```python
from build123d import *

# Parameters (mm, degrees)
F0_W     = 116.948664
F0_H     = 61.326738
F0_W_2   = 104.968556
F0_H_2   = 48.77615
F1_DEPTH = 50.8
F2_W     = 55.336682
F2_H     = 18.995669
F3_DEPTH = 76.2
F4_R     = 6.426074
F5_DEPTH = 177.8


with BuildPart() as f1:
    # F0 (on Top) → F1 (new body)
    with BuildSketch(Plane.XY):
        with Locations((3.137648, -3.137646)):
            Rectangle(F0_W, F0_H)
        with Locations((3.708128, -3.137648)):
            Rectangle(F0_W_2, F0_H_2, mode=Mode.SUBTRACT)
    extrude(amount=F1_DEPTH)

    # F2 (on face) → F3 (cut)
    with BuildSketch(Plane.XZ.offset(33.801015)):
        with Locations((2.281924, 41.302166)):
            Rectangle(F2_W, F2_H)
    extrude(amount=-F3_DEPTH, mode=Mode.SUBTRACT)

    # F4 (on face) → F5 (cut)
    with BuildSketch(Plane.YZ.offset(61.61198)):
        with Locations((-3.137646, 25.4)):
            Circle(F4_R)
    extrude(amount=-F5_DEPTH, mode=Mode.SUBTRACT)


solid = f1.part
```
For this review, take the finished solid that the model builds, in its own axes (mm). A direction names the side the tool comes from. Round coordinates to 2 decimals unless told otherwise and drop trailing zeros. Order: outer loops, then holes, each group sorted by start corner. A loop starts at its lowest first (then second) coordinate and runs counter-clockwise, first axis right, second up.
Q1. Mouldability with a two-part tool opening along Y and no side actions: class faces 4 (the cylindrical face through (58.94, -3.97, 31.77)), 5 (the flat face through (2, -31, 31.804)), 6 (the flat face through (3, -27.526, 19)), 7 (the flat face through (2, -33.801, 19)) as pulls with the +Y half, pulls with the -Y half, needs draft (parallel to the pull), parting line crosses it, or undercut.
Findings below:
face 4: undercut
face 5: needs draft
face 6: undercut
face 7: pulls with the -Y half
Q2. We need section A-A, the plane x = -8. Give the boundary of the cut face in (y, z).
Findings below:
outline: (-33.8, 0) - (-27.53, 0) - (-27.53, 31.8) - (-33.8, 31.8) - close; (21.25, 0) - (27.53, 0) - (27.53, 31.8) - (21.25, 31.8) - close
Q3. Insertion check: P1, Ø7, axis at x = 3.5, y = -31, coming from the +Z side. The pin has a flat end and moves straight along its axis. Give the tip position at first contact, or say it passes through.
Findings below:
P1: stops at z = 31.8
Q4. We need section C-C, the plane y = -2. Give the boundary of the cut face in (x, z), plus the area to 3 significant figures.
Findings below:
outline: (-55.34, 0) - (-48.78, 0) - (-48.78, 19.08) - (-55.34, 19.08) - close; (-55.34, 31.72) - (-48.78, 31.72) - (-48.78, 50.8) - (-55.34, 50.8) - close; (56.19, 0) - (61.61, 0) - (61.61, 19.08) - (56.19, 19.08) - close; (56.19, 31.72) - (61.61, 31.72) - (61.61, 50.8) - (56.19, 50.8) - close
area: 457 mm2
Q5. We need section B-B, the plane z = 35. Give the boundary of the cut face in (x, y), plus the area to 3 significant figures.
Findings below:
outline: (-55.34, -33.8) - (-25.39, -33.8) - (-25.39, -27.53) - (-48.78, -27.53) - (-48.78, 21.25) - (-25.39, 21.25) - (-25.39, 27.53) - (-55.34, 27.53) - close; (29.95, -33.8) - (61.61, -33.8) - (61.61, 27.53) - (29.95, 27.53) - (29.95, 21.25) - (56.19, 21.25) - (56.19, -27.53) - (29.95, -27.53) - close
area: 1,360 mm2
Q6. Wall thickness on line 1 (X direction, y = 24.5, z = 49); line 2 (Y direction, x = -26, z = 38); line 3 (X direction, y = 10, z = 8): over which ranges is each line inside the solid? List them lowest first.
Findings below:
line 1: x = -55.34 to -25.39, 29.95 to 61.61
line 2: y = -33.8 to -27.53, 21.25 to 27.53
line 3: x = -55.34 to -48.78, 56.19 to 61.61
Q7. Machinability: for faces 1 (the flat face through (56.192, -9, 31)), 2 (the flat face through (29.95, -31, 41)), 3 (the flat face through (57, -1, 50.8)), which of the approach directions +Z, -Z, +X, -X, +Y, -Y give a long, thin tool a straight path to every point of the face, cutting with its end or side? Answer none if there is none.
Findings below:
face 1: +Z, -Z
face 2: +Z, +Y, -Y
face 3: +Z, +X, -X, +Y, -Y
Q8. We need section D-D, the plane z = 10.5. Give the boundary of the cut face in (x, y), plus the area to 3 significant figures.
Findings below:
outline: (-55.34, -33.8) - (61.61, -33.8) - (61.61, 27.53) - (-55.34, 27.53) - close; hole (-48.78, -27.53) - (56.19, -27.53) - (56.19, 21.25) - (-48.78, 21.25) - close
area: 2,050 mm2
